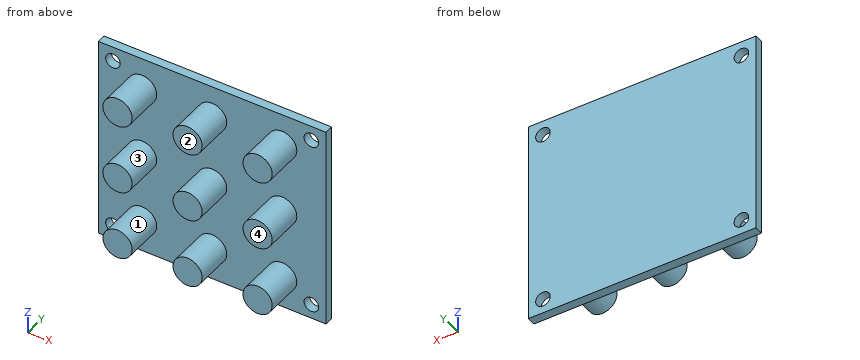
from build123d import *

# Parameters (mm, degrees)
F0_W     = 39
F0_H     = 35
F0_R     = 1.25
F0_R_2   = 2.5
F1_DEPTH = 1.5
F2_DEPTH = 8


with BuildPart() as f1:
    # F0 (on Front) → F1 (new body)
    with BuildSketch(Plane.XZ):
        with Locations((-21.04439, 36.519036)):
            Rectangle(F0_W, F0_H)
        with Locations((-38.04439, 21.519036)):
            Circle(F0_R, mode=Mode.SUBTRACT)
        with Locations((-33.04439, 24.519036)):
            Circle(F0_R_2, mode=Mode.SUBTRACT)
        with Locations((-21.04439, 24.519036)):
            Circle(F0_R_2, mode=Mode.SUBTRACT)
        with Locations((-4.04439, 21.519036)):
            Circle(F0_R, mode=Mode.SUBTRACT)
        with Locations((-9.04439, 24.519036)):
            Circle(F0_R_2, mode=Mode.SUBTRACT)
        with Locations((-33.04439, 36.519036)):
            Circle(F0_R_2, mode=Mode.SUBTRACT)
        with Locations((-21.04439, 36.519036)):
            Circle(F0_R_2, mode=Mode.SUBTRACT)
        with Locations((-33.04439, 48.519036)):
            Circle(F0_R_2, mode=Mode.SUBTRACT)
        with Locations((-38.04439, 51.519036)):
            Circle(F0_R, mode=Mode.SUBTRACT)
        with Locations((-21.04439, 48.519036)):
            Circle(F0_R_2, mode=Mode.SUBTRACT)
        with Locations((-9.04439, 36.519036)):
            Circle(F0_R_2, mode=Mode.SUBTRACT)
        with Locations((-9.04439, 48.519036)):
            Circle(F0_R_2, mode=Mode.SUBTRACT)
        with Locations((-4.04439, 51.519036)):
            Circle(F0_R, mode=Mode.SUBTRACT)
    extrude(amount=F1_DEPTH)

    # F0 (on Front) → F2 (join)
    with BuildSketch(Plane.XZ):
        with Locations((-33.04439, 48.519036)):
            Circle(F0_R_2)
        with Locations((-21.04439, 48.519036)):
            Circle(F0_R_2)
        with Locations((-9.04439, 48.519036)):
            Circle(F0_R_2)
        with Locations((-33.04439, 36.519036)):
            Circle(F0_R_2)
        with Locations((-21.04439, 36.519036)):
            Circle(F0_R_2)
        with Locations((-9.04439, 36.519036)):
            Circle(F0_R_2)
        with Locations((-33.04439, 24.519036)):
            Circle(F0_R_2)
        with Locations((-21.04439, 24.519036)):
            Circle(F0_R_2)
        with Locations((-9.04439, 24.519036)):
            Circle(F0_R_2)
    extrude(amount=F2_DEPTH)


solid = f1.part
Model file for the job. Use its own axes, mm. Face numbers are marked on the shaded views. A direction names the side the tool comes from. Give positions to 0.01 mm unless a question says otherwise; leave off trailing zeros. Loops run counter-clockwise (first coordinate to the right, second up) from the corner with the lowest first, then second, coordinate; pieces in that order, holes last.
Item 1: Drop a flat-ended pin along its axis: P1, Ø1.5, axis at x = -20, z = 30.5, coming from the -Y side. Give the stop position or say it passes through.
Check values:
P1: stops at y = -1.5
Item 2: Which spindle directions (+Z, -Z, +X, -X, +Y, -Y) get a long thin tool onto all of the face, cutting with end or side? Do the marked faces 1 and 2. Say none if no direction does.
Check values:
face 1: -Y
face 2: +Z, -Z, +X, -X, -Y
Item 3: Slice it at D-D (x = -8). Write the cut outline in (y, z), plus the area to 3 significant figures.
Check values:
outline: (-8, 22.25) - (-1.5, 22.25) - (-1.5, 19.02) - (0, 19.02) - (0, 54.02) - (-1.5, 54.02) - (-1.5, 50.79) - (-8, 50.79) - (-8, 46.25) - (-1.5, 46.25) - (-1.5, 38.79) - (-8, 38.79) - (-8, 34.25) - (-1.5, 34.25) - (-1.5, 26.79) - (-8, 26.79) - close
area: 141 mm2
Item 4: Slice it at A-A (y = -4.25). Give the number of separate pieces and of enclosed holes in the cut face, plus the area to 3 significant figures.
Check values:
separate pieces: 9
enclosed holes: 0
area: 177 mm2
Item 5: Mould opens along Z. For the marked faces 3 and 4 say: +Z half, -Z half, draft (parallel to the pull), parting line (faces both ways), or undercut.
Check values:
face 3: undercut
face 4: draft
Item 6: Drill centre lines: line 1 along Z through (x, y) = (-21, -2); line 2 along Z through (x, y) = (-19.5, -1.75); line 3 along Y through (x, z) = (-26, 25). Where is each one in solid material? Low to high.
Check values:
line 1: z = 22.02 to 27.02, 34.02 to 39.02, 46.02 to 51.02
line 2: z = 22.55 to 26.48, 34.55 to 38.48, 46.55 to 50.48
line 3: y = -1.5 to 0
Item 7: Slice it at B-B (x = -38). Write the cut outline in (y, z).
Check values:
outline: (-1.5, 19.02) - (0, 19.02) - (0, 20.27) - (-1.5, 20.27) - close; (-1.5, 22.77) - (0, 22.77) - (0, 50.27) - (-1.5, 50.27) - close; (-1.5, 52.77) - (0, 52.77) - (0, 54.02) - (-1.5, 54.02) - close
Item 8: Slice it at C-C (z = 52). Write the cut outline in (x, y), plus the area to 3 significant figures.
Check values:
outline: (-40.54, -1.5) - (-39.2, -1.5) - (-39.2, 0) - (-40.54, 0) - close; (-36.89, -1.5) - (-5.2, -1.5) - (-5.2, 0) - (-36.89, 0) - close; (-2.89, -1.5) - (-1.54, -1.5) - (-1.54, 0) - (-2.89, 0) - close
area: 51.6 mm2
